```python
from build123d import *

# Parameters (mm, degrees)
SKETCH1_W                                     = 177.8
SKETCH1_H                                     = 311.15
EXTRUDE1_DEPTH                                = 25.4
CBORE_FOR_3_8_SOCKET_HEAD_CAP_SCREW1_AT_COUNT = 2
CBORE_FOR_3_8_SOCKET_HEAD_CAP_SCREW1_AT_PITCH = 142.980794165
CBORE_FOR_3_8_SOCKET_HEAD_CAP_SCREW1_2_COUNT  = 2
CBORE_FOR_3_8_SOCKET_HEAD_CAP_SCREW1_2_PITCH  = 82.55
CBORE_FOR_3_8_SOCKET_HEAD_CAP_SCREW1_3_COUNT  = 2
CBORE_FOR_3_8_SOCKET_HEAD_CAP_SCREW1_3_PITCH  = 142.980794165
CBORE_FOR_3_8_SOCKET_HEAD_CAP_SCREW1_4_COUNT  = 2
CBORE_FOR_3_8_SOCKET_HEAD_CAP_SCREW1_4_PITCH  = 165.1
CBORE_FOR_3_8_SOCKET_HEAD_CAP_SCREW1_5_COUNT  = 2
CBORE_FOR_3_8_SOCKET_HEAD_CAP_SCREW1_5_PITCH  = 82.55
SKETCH4_R                                     = 44.45
CUT_EXTRUDE1_DEPTH                            = 26.4
SKETCH8_R                                     = 63.5
CUT_EXTRUDE4_DEPTH                            = 1.27
SKETCH9_R                                     = 181.94716953
SKETCH9_R_2                                   = 101.6
CUT_EXTRUDE5_DEPTH                            = 1.27
F_1_4_20_TAPPED_HOLE1_AT_2_COUNT              = 2
F_1_4_20_TAPPED_HOLE1_AT_2_PITCH              = 109.985226281
F_1_4_20_TAPPED_HOLE1_AT_3_COUNT              = 2
F_1_4_20_TAPPED_HOLE1_AT_3_PITCH              = 109.985226281
SKETCH18_W                                    = 69.85
SKETCH18_H                                    = 50.8
SKETCH18_W_2                                  = 101.6
CUT_EXTRUDE7_DEPTH                            = 26.4
SKETCH19_W                                    = 38.1
SKETCH19_H                                    = 2.159
SKETCH19_W_2                                  = 177.8
SKETCH19_H_2                                  = 11.684
CUT_EXTRUDE8_DEPTH                            = 26.4
F_1_2_20_TAPPED_HOLE1_AT_2_COUNT              = 2
F_1_2_20_TAPPED_HOLE1_AT_2_PITCH              = 274.589771749
F_1_2_20_TAPPED_HOLE1_AT_3_COUNT              = 2
F_1_2_20_TAPPED_HOLE1_AT_3_PITCH              = 274.589771749
FILLET2_R                                     = 12.7
CHAMFER1_SIZE                                 = 1.27


with BuildPart() as part:
    # Sketch1 → Extrude1 (new body)
    with BuildSketch(Plane(origin=(0, 0, 0), x_dir=(1, 0, 0), z_dir=(0, 1, 0))):
        with Locations((0, 3.175)):
            Rectangle(SKETCH1_W, SKETCH1_H)
    extrude(amount=EXTRUDE1_DEPTH)

    # Sketch2 → CBORE for 3_8 Socket Head Cap Screw1 (revolve, cut)
    with BuildSketch(Plane(origin=(-71.490397082, 25.4, -41.275), x_dir=(0, 0, 1), z_dir=(1, 0, 0))):
        Polygon((0, 0), (0, 25.4), (5.715, 25.4), (5.15874, 24.76009607), (5.15874, 10.16), (7.9375, 10.16), (7.9375, 0), align=None)
    cbore_for_3_8_socket_head_cap_screw1 = revolve(axis=Axis((-71.490397082, 31.75, -41.275), (0, -1, 0)), mode=Mode.SUBTRACT)

    # CBORE for 3_8 Socket Head Cap Screw1 at: CBORE for 3_8 Socket Head Cap Screw1 ×2
    with Locations(*[Vector(0.5, 0, 0.866025404) * (i * CBORE_FOR_3_8_SOCKET_HEAD_CAP_SCREW1_AT_PITCH) for i in range(1, CBORE_FOR_3_8_SOCKET_HEAD_CAP_SCREW1_AT_COUNT)]):
        add(cbore_for_3_8_socket_head_cap_screw1, mode=Mode.SUBTRACT)

    # CBORE for 3_8 Socket Head Cap Screw1 2: CBORE for 3_8 Socket Head Cap Screw1 ×2
    with Locations(*[Vector(0.866025404, 0, -0.5) * (i * CBORE_FOR_3_8_SOCKET_HEAD_CAP_SCREW1_2_PITCH) for i in range(1, CBORE_FOR_3_8_SOCKET_HEAD_CAP_SCREW1_2_COUNT)]):
        add(cbore_for_3_8_socket_head_cap_screw1, mode=Mode.SUBTRACT)

    # CBORE for 3_8 Socket Head Cap Screw1 3: CBORE for 3_8 Socket Head Cap Screw1 ×2
    with Locations(*[(i * CBORE_FOR_3_8_SOCKET_HEAD_CAP_SCREW1_3_PITCH, 0, 0) for i in range(1, CBORE_FOR_3_8_SOCKET_HEAD_CAP_SCREW1_3_COUNT)]):
        add(cbore_for_3_8_socket_head_cap_screw1, mode=Mode.SUBTRACT)

    # CBORE for 3_8 Socket Head Cap Screw1 4: CBORE for 3_8 Socket Head Cap Screw1 ×2
    with Locations(*[Vector(0.866025404, 0, 0.5) * (i * CBORE_FOR_3_8_SOCKET_HEAD_CAP_SCREW1_4_PITCH) for i in range(1, CBORE_FOR_3_8_SOCKET_HEAD_CAP_SCREW1_4_COUNT)]):
        add(cbore_for_3_8_socket_head_cap_screw1, mode=Mode.SUBTRACT)

    # CBORE for 3_8 Socket Head Cap Screw1 5: CBORE for 3_8 Socket Head Cap Screw1 ×2
    with Locations(*[(0, 0, i * CBORE_FOR_3_8_SOCKET_HEAD_CAP_SCREW1_5_PITCH) for i in range(1, CBORE_FOR_3_8_SOCKET_HEAD_CAP_SCREW1_5_COUNT)]):
        add(cbore_for_3_8_socket_head_cap_screw1, mode=Mode.SUBTRACT)

    # Sketch4 → Cut-Extrude1 (cut, through all)
    with BuildSketch(Plane(origin=(0, 25.4, 0), x_dir=(1, 0, 0), z_dir=(0, 1, 0))):
        with Locations(Location((0, 0, 0), (0, 0, 270))):  # turned: the seam where the file's is
            Circle(SKETCH4_R)
    extrude(amount=-CUT_EXTRUDE1_DEPTH, mode=Mode.SUBTRACT)

    # Sketch8 → Cut-Extrude4 (cut)
    with BuildSketch(Plane.XZ):
        with Locations(Location((0, 0, 0), (0, 0, 270))):  # turned: the seam where the file's is
            Circle(SKETCH8_R)
    extrude(amount=-CUT_EXTRUDE4_DEPTH, mode=Mode.SUBTRACT)

    # Sketch9 → Cut-Extrude5 (cut)
    with BuildSketch(Plane.XZ):
        Circle(SKETCH9_R)
        Circle(SKETCH9_R_2, mode=Mode.SUBTRACT)
    extrude(amount=-CUT_EXTRUDE5_DEPTH, mode=Mode.SUBTRACT)

    # Sketch10 → 1_4-20 Tapped Hole1 (revolve, cut)
    with BuildSketch(Plane(origin=(-63.5, 25.4, 0), x_dir=(0, 0, 1), z_dir=(1, 0, 0))):
        Polygon((0, 0), (0, 16.51), (2.5527, 16.51), (2.5527, 12.7), (3.175, 12.7), (3.175, 0.730483939), (3.81, 0), align=None)
    f_1_4_20_tapped_hole1 = revolve(axis=Axis((-63.5, 31.75, 0), (0, -1, 0)), mode=Mode.SUBTRACT)

    # 1_4-20 Tapped Hole1 at 2: 1_4-20 Tapped Hole1 ×2
    with Locations(*[Vector(0.866025404, 0, 0.5) * (i * F_1_4_20_TAPPED_HOLE1_AT_2_PITCH) for i in range(1, F_1_4_20_TAPPED_HOLE1_AT_2_COUNT)]):
        add(f_1_4_20_tapped_hole1, mode=Mode.SUBTRACT)

    # 1_4-20 Tapped Hole1 at 3: 1_4-20 Tapped Hole1 ×2
    with Locations(*[Vector(0.866025404, 0, -0.5) * (i * F_1_4_20_TAPPED_HOLE1_AT_3_PITCH) for i in range(1, F_1_4_20_TAPPED_HOLE1_AT_3_COUNT)]):
        add(f_1_4_20_tapped_hole1, mode=Mode.SUBTRACT)

    # Sketch18 → Cut-Extrude7 (cut, through all)
    with BuildSketch(Plane(origin=(0, 25.4, 0), x_dir=(1, 0, 0), z_dir=(0, 1, 0))):
        with Locations((53.975, 133.35)):
            Rectangle(SKETCH18_W, SKETCH18_H)
        with Locations((-53.975, 133.35)):
            Rectangle(SKETCH18_W, SKETCH18_H)
        with Locations((0, -127)):
            Rectangle(SKETCH18_W_2, SKETCH18_H)
    extrude(amount=-CUT_EXTRUDE7_DEPTH, mode=Mode.SUBTRACT)

    # Sketch19 → Cut-Extrude8 (cut, through all)
    with BuildSketch(Plane(origin=(0, 25.4, 0), x_dir=(1, 0, 0), z_dir=(0, 1, 0))):
        with Locations((0, 157.6705)):
            Rectangle(SKETCH19_W, SKETCH19_H)
        with Locations((0, -146.558)):
            Rectangle(SKETCH19_W_2, SKETCH19_H_2)
    extrude(amount=-CUT_EXTRUDE8_DEPTH, mode=Mode.SUBTRACT)

    # Sketch14 → 1_2-20 Tapped Hole1 (revolve, cut)
    with BuildSketch(Plane(origin=(0, 25.4, -140.716), x_dir=(0, 0, 1), z_dir=(1, 0, 0))):
        Polygon((0, 0), (0, 24.13), (6.985, 24.13), (5.75437, 22.714322127), (5.75437, 1.415677873), (6.985, 0), align=None)
    f_1_2_20_tapped_hole1 = revolve(axis=Axis((0, 31.75, -140.716), (0, -1, 0)), mode=Mode.SUBTRACT)

    # 1_2-20 Tapped Hole1 at 2: 1_2-20 Tapped Hole1 ×2
    with Locations(*[Vector(0.254379468, 0, 0.967104486) * (i * F_1_2_20_TAPPED_HOLE1_AT_2_PITCH) for i in range(1, F_1_2_20_TAPPED_HOLE1_AT_2_COUNT)]):
        add(f_1_2_20_tapped_hole1, mode=Mode.SUBTRACT)

    # 1_2-20 Tapped Hole1 at 3: 1_2-20 Tapped Hole1 ×2
    with Locations(*[Vector(-0.254379468, 0, 0.967104486) * (i * F_1_2_20_TAPPED_HOLE1_AT_3_PITCH) for i in range(1, F_1_2_20_TAPPED_HOLE1_AT_3_COUNT)]):
        add(f_1_2_20_tapped_hole1, mode=Mode.SUBTRACT)

    # Fillet2
    fillet2_edges = [part.edges().sort_by_distance(p)[0] for p in [
        (19.05, 13.335, -107.95),
        (-19.05, 13.335, -107.95),
        (-50.8, 13.335, 101.6),
        (50.8, 13.335, 101.6),
    ]]
    fillet(fillet2_edges, radius=FILLET2_R)

    # Chamfer1
    chamfer1_edges = [part.edges().sort_by_distance(p)[0] for p in [
        (88.9, 13.335, -107.95),
        (-88.9, 13.335, -107.95),
        (-19.05, 13.335, -156.591),
        (19.05, 13.335, -156.591),
        (50.8, 13.335, 140.716),
        (-88.9, 13.335, 140.716),
        (-50.8, 13.335, 140.716),
        (88.9, 13.335, 140.716),
    ]]
    chamfer(chamfer1_edges, length=CHAMFER1_SIZE)


solid = part.part
```
For this review, take the finished solid that the model builds, in its own axes (mm). A direction names the side the tool comes from. Round coordinates to 2 decimals unless told otherwise and drop trailing zeros. Write each loop counter-clockwise with the first axis right and the second up, starting at its lowest first coordinate (ties: lowest second). Pieces come first, ordered by that corner, then holes. Notation, with made-up numbers: M 66.25,73 L 77.25,73 A18 cw 77.25,77 Z; hole C 70,70 d2. An arc over 180 degrees is marked long. One line per item, written item: value. Start each with the question number.
(1) The part is to be moulded in two halves that separate along Z. For faces 5 (the flat face through (0, 14, -156.591)), 6 (the cylindrical face through (4.577, 8.042, -80.17)), 7 (the flat face through (67, 1.27, 102)), say which applies: released by +Z, released by -Z, zero draft, split by the parting line, or undercut.
(2) We need section C-C (y = 21). Count the separate pieces of the cut face and the enclosed holes in it, and give its area (3 significant figures).
(3) We need section A-A (z = -9.5). Give the boundary of the cut face in (x, y), and give its area (3 significant figures).
(4) Insertion check: pin 1 (5 mm diameter, centred on x = 31.75, z = -54.99, fed in from +Y); pin 2 (10 mm diameter, centred on x = 44, y = 3.5, fed in from +Z); pin 3 (12.5 mm diameter, centred on x = 72.5, z = 40.5, fed in from +Y); pin 4 (12 mm diameter, centred on y = 7.5, z = -112, fed in from +X). Each pin has a flat end and moves straight along its axis. Give the tip position at first contact, or say it passes through.
(5) We need section B-B (z = -82.55). Give the boundary of the cut face in (x, y) (1 decimal).
(6) Machinability: for faces 1 (the cylindrical face through (-73.74, 13.48, 120.6)), 2 (the cylindrical face through (-2.384, 20.391, 90.121)), 3 (the flat face through (-50.8, 14, 127)), 4 (the flat face through (59, 14, -107.95)), which of the approach directions +Z, -Z, +X, -X, +Y, -Y give a long, thin tool a straight path to every point of the face, cutting with its end or side? Answer none if there is none.
(7) Wall thickness on line 1 (X direction, y = 9.7, z = 0); line 2 (Z direction, x = -77, y = 20); line 3 (Z direction, x = 33.5, y = 10.25): over which ranges is each line inside the solid? List them lowest first.
Result:
1. face 5: released by -Z
1. face 6: undercut
1. face 7: zero draft
2. separate pieces: 1
2. enclosed holes: 13
2. area: 34,400 mm²
3. outline: M -88.9,0 L -62.79,0 L -62.79,1.27 L -43.42,1.27 L -43.42,25.4 L -88.9,25.4 Z; M 43.42,1.27 L 62.79,1.27 L 62.79,0 L 88.9,0 L 88.9,25.4 L 43.42,25.4 Z
3. area: 2,260 mm²
4. pin 1: y = 8.89
4. pin 2: z = 107.78
4. pin 3: y = 15.24
4. pin 4: x = 88.9
5. outline: M -88.9,1.3 L -59.2,1.3 L -59.2,0 L -5.7,0 L -5.2,0.6 L -5.2,15.2 L -7.9,15.2 L -7.9,25.4 L -88.9,25.4 Z; M 5.2,0.6 L 5.7,0 L 59.2,0 L 59.2,1.3 L 88.9,1.3 L 88.9,25.4 L 7.9,25.4 L 7.9,15.2 L 5.2,15.2 Z
6. face 1: +Y, -Y
6. face 2: +Y
6. face 3: +Z, +Y, -Y
6. face 4: -Z, +X, +Y, -Y
7. line 1: -88.9 to -66.05, -60.95 to -44.45, 44.45 to 88.9
7. line 2: -107.95 to -46.99, -35.56 to 35.56, 46.99 to 140.72
7. line 3: -107.95 to -56.85, -53.13 to -29.22, 29.22 to 53.13, 56.85 to 101.6
